Can you work these out from the model? Positions are in its coordinate system, mm. A direction names the side the tool comes from. Give positions to 0.01 mm unless a question says otherwise; leave off trailing zeros. Order: outer loops, then holes, each group sorted by start corner. A loop starts at its lowest first (then second) coordinate and runs counter-clockwise, first axis right, second up. Notation, with made-up numbers: M -9.5,3 L 4.5,3 A19 ccw 4.5,10 Z; hole C 83,64 d11. An arc over 180 degrees is marked long. Answer as a JSON object with one key per item and string values.
```python
from build123d import *

# Parameters (mm, degrees)
F_3_8_0_375_DIAMETER_HOLE1_D     = 9.525
F_3_8_0_375_DIAMETER_HOLE1_DEPTH = 77.7875
F_3_8_0_375_DIAMETER_HOLE1_TIP   = 2.861598698
CHAMFER1_SIZE                    = 1.5875


with BuildPart() as part:
    # Sketch1 → Revolve1 (revolve)
    with BuildSketch(Plane.XY):
        Polygon((0, 0), (-19.05, 0), (-19.05, -6.35), (-17.4625, -6.35), (-17.4625, -3.81), (-14.1605, -3.81), (-14.1605, -6.35), (-6.35, -6.35), (-6.35, -82.55), (0, -82.55), align=None)
    revolve(axis=Axis((0, -82.55, 0), (0, 1, 0)))

    # 3/8 (0.375) Diameter Hole1
    with Locations(Plane(origin=(0, 0, 0), x_dir=(1, 0, 0), z_dir=(0, 1, 0))):
        with Locations((0, 0)):
            Hole(F_3_8_0_375_DIAMETER_HOLE1_D / 2, depth=F_3_8_0_375_DIAMETER_HOLE1_DEPTH)
            with Locations((0, 0, -(F_3_8_0_375_DIAMETER_HOLE1_DEPTH + F_3_8_0_375_DIAMETER_HOLE1_TIP / 2))):  # 118° drill point
                Cone(0, F_3_8_0_375_DIAMETER_HOLE1_D / 2, F_3_8_0_375_DIAMETER_HOLE1_TIP, mode=Mode.SUBTRACT)

    # Chamfer1
    chamfer1_edges = [part.edges().sort_by_distance(p)[0] for p in [
        (6.35, -82.55, 0),
    ]]
    chamfer(chamfer1_edges, length=CHAMFER1_SIZE)


solid = part.part
```
1) I want a section at C-C on x = 15. Write out the boundary of the cut face in (y, z), and give its area (3 significant figures).
Results found:
{"outline": "M -6.35,-11.74 L 0,-11.74 L 0,11.74 L -6.35,11.74 L -6.35,8.94 L -3.81,8.94 L -3.81,-8.94 L -6.35,-8.94 Z", "area": "104 mm²"}
2) For faces 4 (the face through (-3, -6.35, -6)), 5 (the face through (0, -82.55, 0)), 6 (the face through (3.78, -39.44, 2.9)), which set-ups out of +Z, -Z, +X, -X, +Y, -Y let a thin tool reach every point of the face, with its end or its side?
Results found:
{"face 4": "-Y", "face 5": "+Z, -Z, +X, -X, -Y", "face 6": "+Y"}
3) I want a section at D-D on z = -9.5. Write out the boundary of the cut face in (x, y), and give its area (3 significant figures).
Results found:
{"outline": "M -16.51,-6.35 L -14.65,-6.35 L -14.65,-3.81 L -10.5,-3.81 L -10.5,-6.35 L 10.5,-6.35 L 10.5,-3.81 L 14.65,-3.81 L 14.65,-6.35 L 16.51,-6.35 L 16.51,0 L -16.51,0 Z", "area": "189 mm²"}
4) I'm going to push flat-ended pins straight in: pin 1 Ø12 at (x, y) = (-1.5, -63.5) entering from -Z; pin 2 Ø10 at (x, y) = (10.5, -15.5) entering from +Z; pin 3 Ø1.5 at (x, z) = (2.5, -5.5) entering from -Y; pin 4 Ø8 at (x, y) = (14, -23.5) entering from +Z. Where does each tip first touch, or does it pass through?
Results found:
{"pin 1": "stops at z = -6.35", "pin 2": "stops at z = 3.17", "pin 3": "stops at y = -82.02", "pin 4": "passes through"}
5) Thinking about a two-plate mould opening in Z: for faces 1 (the face through (1.84, -5.1, 14.04)), 2 (the face through (-17, -6.35, -6)), 3 (the face through (15.12, -3.22, -11.59)), which applies, pulls with the +Z half, pulls with the -Z half, needs draft (parallel to the pull), parting line crosses it, or undercut?
Results found:
{"face 1": "undercut", "face 2": "needs draft", "face 3": "parting line crosses it"}
6) I want a section at A-A on z = 11.5. Write out the boundary of the cut face in (x, y), and give its area (3 significant figures).
Results found:
{"outline": "M -15.19,-6.35 L -13.14,-6.35 L -13.14,-3.81 L -8.26,-3.81 L -8.26,-6.35 L 8.26,-6.35 L 8.26,-3.81 L 13.14,-3.81 L 13.14,-6.35 L 15.19,-6.35 L 15.19,0 L -15.19,0 Z", "area": "168 mm²"}
7) I need wall thicknesses on L1, parallel to Z at x = 0, y = -23.5; L2, parallel to Z at x = -4, y = -10; L3, parallel to Y at x = -9, z = 14.5. Which ranges of each line are inside material? Lowest first, please.
Results found:
{"L1": "z = -6.35 to -4.76, 4.76 to 6.35", "L2": "z = -4.93 to -2.58, 2.58 to 4.93", "L3": "y = -3.81 to 0"}
